Design review of the part shown in the three views and the two pictorial views. Dimensions are in mm from the part's minimum x, y and z. A direction names the side the tool comes from. Coordinates: 2 decimals unless noted, no trailing zeros. Loops run counter-clockwise (first coordinate to the right, second up) from the corner with the lowest first, then second, coordinate; pieces in that order, holes last. Notation, with made-up numbers: (-3, 19.5) - (51, 19.5) arc R27 cw to (51, 38.5) - close; hole circle Ø4 at (2.25, 1). An arc over 180 degrees is marked (long way). One line per question, with ' | ' between items.
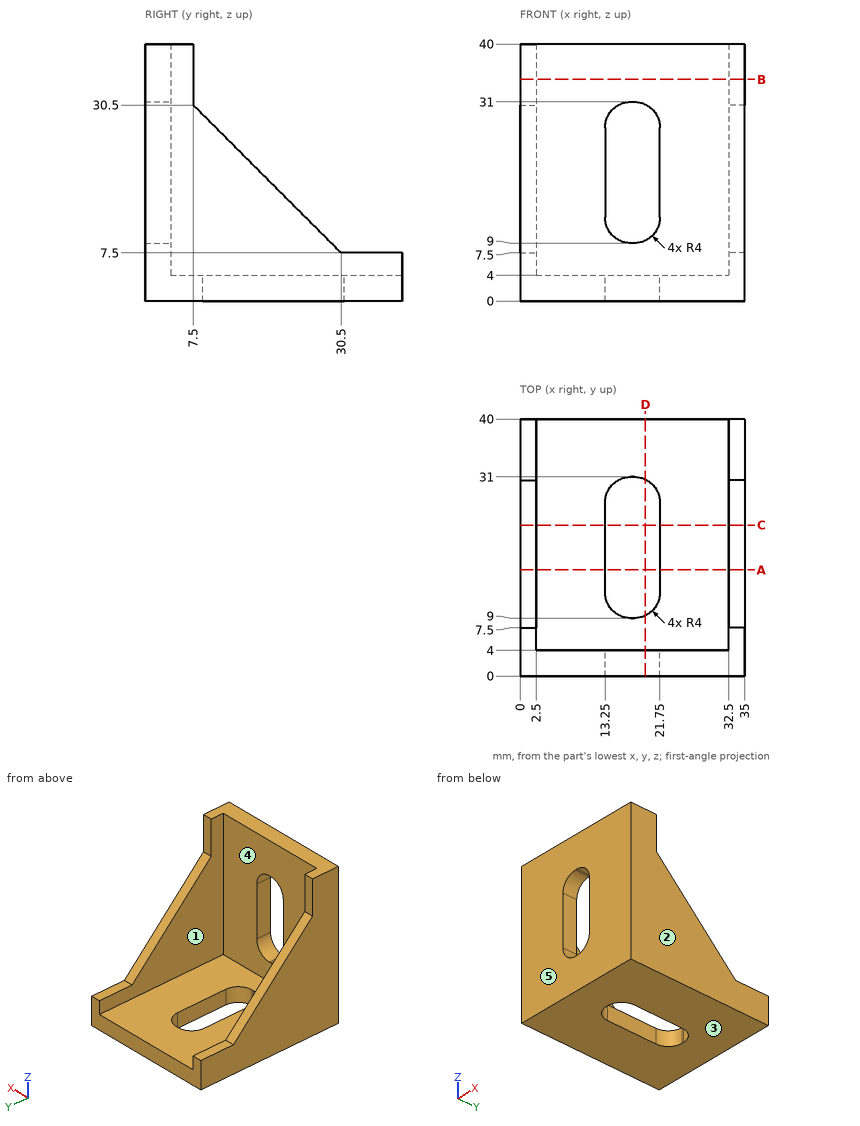
Q1. Take a section at B-B (z = 34.5). Give the boundary of the cut face in (x, y), plus the area to 4 significant figures.
Returned:
outline: (0, 0) - (35, 0) - (35, 7.5) - (32.5, 7.5) - (32.5, 4) - (2.5, 4) - (2.5, 7.5) - (0, 7.5) - close | area: 157.5 mm²
Q2. Tool access review of the marked faces 4 and 5: name each direction out of +Z, -Z, +X, -X, +Y, -Y from which nothing blocks a thin tool from reaching the whole face with its end or side.
Returned:
face 4: +Z, +Y | face 5: +Z, -Z, +X, -X, -Y
Q3. Take a section at C-C (y = 23.5). Give the boundary of the cut face in (x, z), plus the area to 4 significant figures.
Returned:
outline: (0, 0) - (13.25, 0) - (13.25, 4) - (2.5, 4) - (2.5, 14.5) - (0, 14.5) - close; (21.75, 0) - (35, 0) - (35, 14.5) - (32.5, 14.5) - (32.5, 4) - (21.75, 4) - close | area: 158.5 mm²
Q4. Draft analysis for pull direction X (two halves, no side actions). For the marked faces 1, 2 and 3, state which applies: +X half, -X half, draft (parallel to the pull), parting line (faces both ways), or undercut.
Returned:
face 1: undercut | face 2: +X half | face 3: draft
Q5. To check wall thickness, follow line 1 along X through (y, z) = (9, 7.5); line 2 along Y through (x, z) = (27, 8.5). State the ranges of each line that lie inside material, in increasing order.
Returned:
line 1: x = 0 to 2.5, 32.5 to 35 | line 2: y = 0 to 4
Q6. Take a section at A-A (y = 16.5). Give the boundary of the cut face in (x, z), plus the area to 4 significant figures.
Returned:
outline: (0, 0) - (13.25, 0) - (13.25, 4) - (2.5, 4) - (2.5, 21.5) - (0, 21.5) - close; (21.75, 0) - (35, 0) - (35, 21.5) - (32.5, 21.5) - (32.5, 4) - (21.75, 4) - close | area: 193.5 mm²
Q7. For pin 1 (8 mm diameter, centred on x = 15, z = 30.5, fed in from +Y); pin 2 (2 mm diameter, centred on x = 33.5, y = 37.5, fed in from +Z); pin 3 (2 mm diameter, centred on x = 12, y = 19.5, fed in from +Z); pin 4 (5 mm diameter, centred on y = 12, z = 36, fed in from +X), all flat-tipped, find the tip position at first contact; note any pin that passes through.
Returned:
pin 1: stops at y = 4 | pin 2: stops at z = 7.5 | pin 3: stops at z = 4 | pin 4: passes through
Q8. Take a section at D-D (x = 19.5). Give the boundary of the cut face in (y, z), plus the area to 3 significant figures.
Returned:
outline: (0, 0) - (9.4, 0) - (9.4, 4) - (4, 4) - (4, 9.4) - (0, 9.4) - close; (0, 30.6) - (4, 30.6) - (4, 40) - (0, 40) - close; (30.6, 0) - (40, 0) - (40, 4) - (30.6, 4) - close | area: 134 mm²
